```python
from build123d import *

# Parameters (mm, degrees)
CYLINDER044_R           = 3.2
CYLINDER044_DEPTH       = 156
CYLINDER044_ROLL_ANGLE  = 90
CYLINDER042_R           = 1.2
CYLINDER042_DEPTH       = 10
CYLINDER042_PITCH_ANGLE = 90
BOX028_W                = 3
BOX028_H                = 10
BOX028_DEPTH            = 8
BOX027_W                = 13
BOX027_H                = 10
BOX027_DEPTH            = 13
FILLET_R                = 3
FILLET001_R             = 1.5


with BuildPart() as cylinder044:
    # Cylinder044 → Cylinder044 (new body)
    with BuildSketch(Plane.XY):
        Circle(CYLINDER044_R)
    extrude(amount=CYLINDER044_DEPTH)


with BuildPart() as cylinder044_1:
    # Cylinder044 roll: moved
    add(cylinder044.part.rotate(Axis((0, 0, 0), (1, 0, 0)), CYLINDER044_ROLL_ANGLE))


with BuildPart() as cylinder044_2:
    # Cylinder044 placement: moved
    add(cylinder044_1.part.moved(Location((504, 118, 100))))


with BuildPart() as cylinder042:
    # Cylinder042 → Cylinder042 (new body)
    with BuildSketch(Plane.XY):
        Circle(CYLINDER042_R)
    extrude(amount=CYLINDER042_DEPTH)


with BuildPart() as cylinder042_1:
    # Cylinder042 pitch: moved
    add(cylinder042.part.rotate(Axis((0, 0, 0), (0, 1, 0)), CYLINDER042_PITCH_ANGLE))


with BuildPart() as cylinder042_2:
    # Cylinder042 placement: moved
    add(cylinder042_1.part.moved(Location((499, -33, 95))))


with BuildPart() as box028:
    # Box028 → Box028 (new body)
    with BuildSketch(Plane(origin=(499, -38, 92), x_dir=(1, 0, 0), z_dir=(0, 0, 1))):
        with Locations((1.5, 5)):
            Rectangle(BOX028_W, BOX028_H)
    extrude(amount=BOX028_DEPTH)


with BuildPart() as cut018:
    # Box027 → Box027 (new body)
    with BuildSketch(Plane(origin=(499, -38, 92), x_dir=(1, 0, 0), z_dir=(0, 0, 1))):
        with Locations((6.5, 5)):
            Rectangle(BOX027_W, BOX027_H)
    extrude(amount=BOX027_DEPTH)

    # Fillet
    fillet_edges = [cut018.edges().sort_by_distance(p)[0] for p in [
        (499, -33, 105),
        (512, -33, 105),
    ]]
    fillet(fillet_edges, radius=FILLET_R)

    # Fillet001
    fillet001_edges = [cut018.edges().sort_by_distance(p)[0] for p in [
        (512, -33, 92),
    ]]
    fillet(fillet001_edges, radius=FILLET001_R)

    # Cut016: cut Box028
    add(box028.part, mode=Mode.SUBTRACT)


with BuildPart() as cut018_1:
    # Cut016 placement: moved
    add(cut018.part.moved(Location((-3, 0, 0))))

    # Cut017: cut Cylinder042
    add(cylinder042_2.part, mode=Mode.SUBTRACT)

    # Cut018: cut Cylinder044
    add(cylinder044_2.part, mode=Mode.SUBTRACT)


solid = cut018_1.part
```
For this review, take the finished solid that the model builds, in its own axes (mm). Coordinates: 2 decimals unless noted, no trailing zeros. Loops run counter-clockwise (first coordinate to the right, second up) from the corner with the lowest first, then second, coordinate; pieces in that order, holes last.
1. Add section D-D, the plane y = -36. Give the boundary of the cut face in (x, z), then the cut area to 3 significant figures.
2. Insertion check: P1, Ø2, axis at x = 498.5, y = -30, coming from the +Z side; P2, Ø3, axis at y = -33, z = 95, coming from the -X side. Each pin has a flat end and moves straight along its axis. Give the tip position at first contact, or say it passes through.
3. Add section A-A, the plane x = 504. Give the boundary of the cut face in (y, z).
4. Add section C-C, the plane z = 95. Give the boundary of the cut face in (x, y).
5. Mouldability with a two-part tool opening along Z and no side actions: class faces 1 (the flat face through (499, -33, 97)), 2 (the cylindrical face through (503.93, -32.189, 95.884)), 3 (the flat face through (497, -33, 100)) as +Z half, -Z half, draft (parallel to the pull), parting line (faces both ways), or undercut.
6. Add section B-B, the plane y = -33. Give the boundary of the cut face in (x, z), then the cut area to 3 significant figures.
7. For line 1 (Y direction, x = 503, z = 95); line 2 (Z direction, x = 504, y = -30.75); line 3 (Z direction, x = 505.25, y = -33.25), list the stretches that pass through material, from the lowest coordinate up.
Result:
1. outline: (496, 100) - (499, 100) - (499, 92) - (507.5, 92) arc R1.5 ccw to (509, 93.5) - (509, 102) arc R3 ccw to (506, 105) - (499, 105) arc R3 ccw to (496, 102) - close; hole circle Ø6.4 at (504, 100)
1. area: 108 mm2
2. P1: stops at z = 105
2. P2: stops at x = 499
3. outline: (-38, 92) - (-28, 92) - (-28, 96.8) - (-38, 96.8) - close; (-38, 103.2) - (-28, 103.2) - (-28, 105) - (-38, 105) - close; hole circle Ø2.4 at (-33, 95)
4. outline: (499, -38) - (509, -38) - (509, -34.2) - (499, -34.2) - close; (499, -31.8) - (509, -31.8) - (509, -28) - (499, -28) - close
5. face 1: draft
5. face 2: undercut
5. face 3: -Z half
6. outline: (496, 100) - (499, 100) - (499, 96.2) - (509, 96.2) - (509, 102) arc R3 ccw to (506, 105) - (499, 105) arc R3 ccw to (496, 102) - close; (499, 92) - (507.5, 92) arc R1.5 ccw to (509, 93.5) - (509, 93.8) - (499, 93.8) - close; hole circle Ø6.4 at (504, 100)
6. area: 84.5 mm2
7. line 1: y = -38 to -34.2, -31.8 to -28
7. line 2: z = 92 to 96.8, 103.2 to 105
7. line 3: z = 92 to 93.83, 96.17 to 97.05, 102.95 to 105
